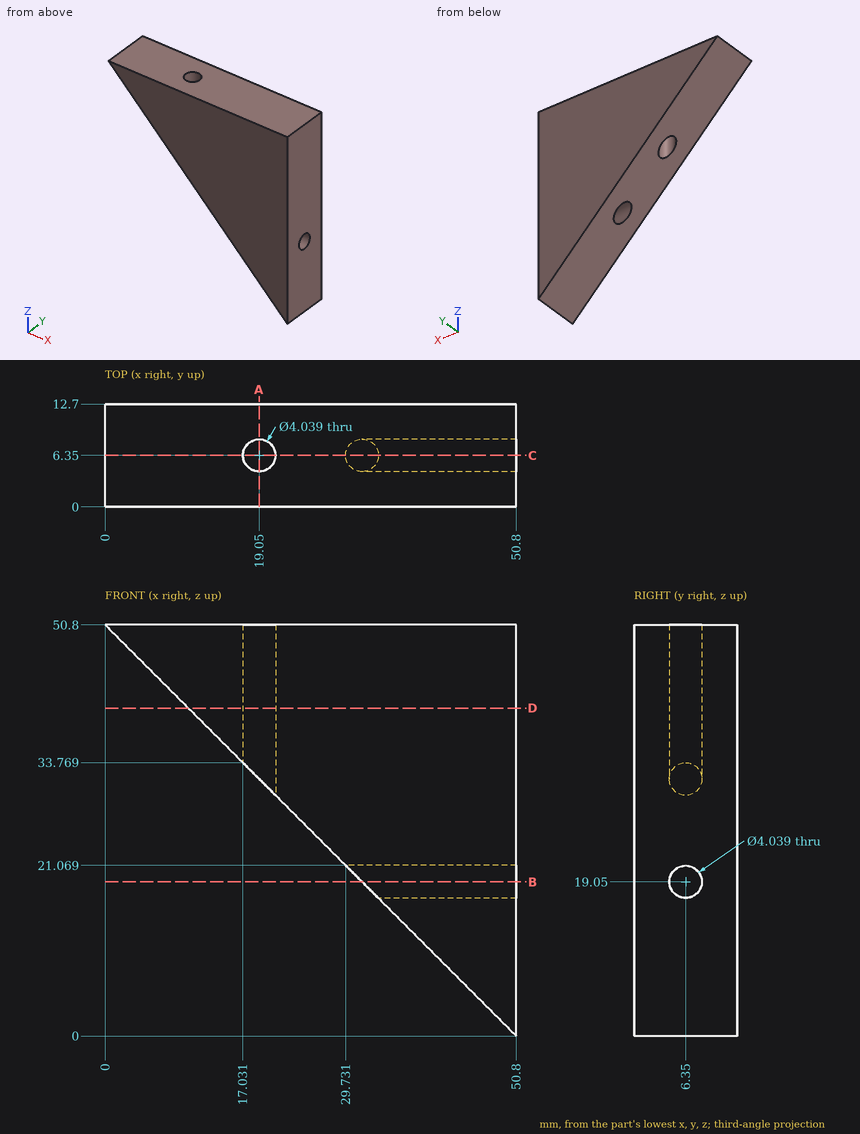
Geometry: see drawing. Coordinates: mm, zero at the bounding-box minimum. Coordinates: 2 decimals unless noted, no trailing zeros. Order: outer loops, then holes, each group sorted by start corner. A loop starts at its lowest first (then second) coordinate and runs counter-clockwise, first axis right, second up. Notation, with made-up numbers: (48, -37.75) - (92, -37.75) arc R15 cw to (92, -27.75) - close; hole circle Ø6 at (-7, -32.75). An arc over 180 degrees is marked (long way). Return JSON: item names as keys, results as strings.
Q1. Cut plane D-D (z = 40.5). Return loops of the section in (x, y).
The answers:
{"outline": "(10.3, 0) - (50.8, 0) - (50.8, 12.7) - (10.3, 12.7) - close; hole circle Ø4.04 at (19.05, 6.35)"}
Q2. Cut plane B-B (z = 19.05). Return loops of the section in (x, y).
The answers:
{"outline": "(31.75, 0) - (50.8, 0) - (50.8, 4.33) - (31.75, 4.33) - close; (31.75, 8.37) - (50.8, 8.37) - (50.8, 12.7) - (31.75, 12.7) - close"}
Q3. Cut plane A-A (x = 19.05). Return loops of the section in (y, z), then the cut area to 3 significant figures.
The answers:
{"outline": "(0, 31.75) - (4.33, 31.75) - (4.33, 50.8) - (0, 50.8) - close; (8.37, 31.75) - (12.7, 31.75) - (12.7, 50.8) - (8.37, 50.8) - close", "area": "165 mm2"}
Q4. Cut plane C-C (y = 6.35). Return loops of the section in (x, z).
The answers:
{"outline": "(0, 50.8) - (17.03, 33.77) - (17.03, 50.8) - close; (21.07, 29.73) - (29.73, 21.07) - (50.8, 21.07) - (50.8, 50.8) - (21.07, 50.8) - close; (33.77, 17.03) - (50.8, 0) - (50.8, 17.03) - close"}
Q5. First-contact query: pin 1 (2 mm diameter, centred on x = 18.5, z = 30.5, fed in from -Y); pin 2 (3 mm diameter, centred on y = 4, z = 28, fed in from -X); pin 3 (4 mm diameter, centred on y = 11, z = 24, fed in from -X). Flat tips, straight axial feed; report the tip coordinate or a pass-through.
The answers:
{"pin 1": "passes through", "pin 2": "stops at x = 21.3", "pin 3": "stops at x = 24.8"}
Q6. Ray query, probe 1 along Y at (x, z) = (34.5, 19.05); probe 2 along Z at (x, y) = (38.75, 6.35); probe 3 along Z at (x, y) = (45, 6.5) (1 decimal). Return the intervals inside material, ascending.
The answers:
{"probe 1": "y = 0 to 4.33, 8.37 to 12.7", "probe 2": "z = 12.05 to 17.03, 21.07 to 50.8", "probe 3": "z = 5.8 to 17, 21.1 to 50.8"}
